Autodesk Inventor part; units mm, degrees
ref_plane "YZ Plane" through (0, 0, 0) normal (1, 0, 0) x (0, 1, 0)
ref_plane "XZ Plane" through (0, 0, 0) normal (0, 1, 0) x (-1, 0, 0)
ref_plane "XY Plane" through (0, 0, 0) normal (0, 0, 1) x (1, 0, 0)
sketch "Sketch_1" plane through (0, 0, 0) normal (0, 0, 1) x (1, 0, 0)
  line L0 (24, 0) -> (0, 0)
  line L1 (0, 0) -> (0, 17.5)
  line L2 (0, 17.5) -> (0.5, 18)
  line L3 (0.5, 18) -> (4.5, 18)
  line L4 (4.5, 18) -> (5, 17.5)
  line L5 (5, 17.5) -> (5, 10.5)
  arc A0 (5, 10.5) -> (5.5, 10) centre (5.5, 10.5) ccw
  line L6 (5.5, 10) -> (23.5, 10)
  line L7 (23.5, 10) -> (24, 9.5)
  line L8 (24, 9.5) -> (24, 0)
  line L9 (24, 0) -> (0, 0)
revolve "Revolution1" add sketch "Sketch_1" angle 360 about axis through (24, 0, 0) along (1, 0, 0)
sketch "Sketch_2" plane through (0, 0, 0) normal (0, 0, 1) x (1, 0, 0)
  line L0 (24, 0) -> (0, 0)
  line L1 (0, 0) -> (0, 5)
  line L2 (0, 5) -> (1, 4)
  line L3 (1, 4) -> (23, 4)
  line L4 (23, 4) -> (24, 5)
  line L5 (24, 5) -> (24, 0)
  line L6 (24, 0) -> (0, 0)
revolve "Revolution2" cut sketch "Sketch_2" angle 360 about axis through (24, 0, 0) along (1, 0, 0)
thread "Thread1"
sketch "Sketch_3" plane through (0, 0, 0) normal (0, 0, 1) x (1, 0, 0)
  line L0 (5, 13) -> (0, 13)
  line L1 (0, 13) -> (0, 15.15)
  line L2 (0, 15.15) -> (5, 15.15)
  line L3 (5, 15.15) -> (5, 13)
  line L4 (5, 13) -> (0, 13)
revolve "Revolution3" cut sketch "Sketch_3" angle 360 about axis through (5, 13, 0) along (1, 0, 0)
pattern_linear "Rectangular Pattern1" count 2 spacing 18.3848 along (0, -0.7071, 0.7071) count 2 spacing 18.3848 along (0, -0.7071, -0.7071) of "Revolution3"
properties part number "MTSRR10"
Build history of the part. All positions in model axes, mm. A direction names the side the tool comes from. Round coordinates to 2 decimals unless told otherwise and drop trailing zeros. Write each loop counter-clockwise with the first axis right and the second up, starting at its lowest first coordinate (ties: lowest second). Pieces come first, ordered by that corner, then holes. Notation, with made-up numbers: (-0.5, 1.25) - (30.5, 1.25) arc R23 ccw to (30.5, 12.25) - close; hole circle Ø8 at (36.5, 69). An arc over 180 degrees is marked (long way). Use CSV: the item, a comma, the result in double quotes.
(1) Band-saw the part on C-C (x = 10). Write the cut outline in (y, z).
Response:
outline,"circle Ø20 at (0, 0); hole circle Ø8 at (0, 0)"
(2) Band-saw the part on A-A (z = 0). Give the number of separate pieces and of enclosed holes in the cut face, plus the area to 3 significant figures.
Response:
separate pieces,"4"
enclosed holes,"0"
area,"322 mm²"
(3) 3-axis set-ups, long thin cutter, end or side, ignore diameter. For faces 1 (the flat face through (5, 8, -8)), 2 (the cylindrical face through (2.54, -10.95, 0.65)): which of +Z, -Z, +X, -X, +Y, -Y reach the whole face in a straight line?
Response:
face 1,"+X"
face 2,"+X, -X"
(4) Wall check: line 1 (X direction, y = 15, z = 1); line 2 (Z direction, x = 20.75, y = 2.5); line 3 (Z direction, x = 7.5, y = -1.5). Give the ranges that are in metal, low to high.
Response:
line 1,"0 to 5"
line 2,"-9.68 to -3.12, 3.12 to 9.68"
line 3,"-9.89 to -3.71, 3.71 to 9.89"
(5) Mould opens along Y. For faces 3 (the flat face through (24, 4, -4)), 4 (the cylindrical face through (14.63, -2.17, -9.76)), 5 (the cylindrical face through (2.54, 15.05, 0.65)) say: pulls with the +Y half, pulls with the -Y half, needs draft (parallel to the pull), parting line crosses it, or undercut.
Response:
face 3,"needs draft"
face 4,"parting line crosses it"
face 5,"undercut"
(6) Pin check, flat tips, straight feed: P1, Ø2, axis at x = 2.5, z = 4.5, coming from the -Y side; P2, Ø5.5, axis at y = 13, z = 0, coming from the +X side; P3, Ø4, axis at x = 20.5, y = 3, coming from the -Z side. Stop position of each tip, or through.
Response:
P1,"y = -17.66"
P2,"x = 5.07"
P3,"z = -9.95"
